```python
from build123d import *

# Parameters (mm, degrees)
F0_W     = 330.2
F0_H     = 533.4
F0_W_2   = 279.4
F0_H_2   = 482.6
F1_DEPTH = 381
F3_DEPTH = 11.43
F5_D     = 31.75
F6_W     = 330.2
F6_H     = 533.4
F7_DEPTH = 25.4


with BuildPart() as f1:
    # F0 (on Front) → F1 (new body)
    with BuildSketch(Plane.XZ):
        Rectangle(F0_W, F0_H)
        Rectangle(F0_W_2, F0_H_2, mode=Mode.SUBTRACT)
    extrude(amount=F1_DEPTH)

    # F2 (on face) → F3 (join)
    with BuildSketch(Plane.YZ.offset(165.1)):
        with BuildLine():
            add(Edge.make_bspline(
                [(-381, -6.6830463366), (-397.4427610563, -10.9233558088), (-440.2612759163, -2.0870202582), (-482.6984064218, 23.1422229449), (-443.5296874883, 46.3759759497), (-397.7583791554, 55.5903688255), (-381, 53.9625514371)],
                knots=[0.054305568, 0.054305568, 0.054305568, 0.054305568, 0.2287997299, 0.4012099815, 0.5729439025, 0.7296806034, 0.7296806034, 0.7296806034, 0.7296806034], degree=3))
            Line((-381, -6.6830463366), (-381, 53.9625514371))
        make_face()
        with BuildLine():
            add(Edge.make_bspline(
                [(-367.3923313618, 0), (-371.2589549432, -3.2025358081), (-375.8827314956, -5.3633894957), (-381, -6.6830463366)],
                knots=[0, 0, 0, 0, 0.054305568, 0.054305568, 0.054305568, 0.054305568], degree=3))
            add(Edge.make_bspline(
                [(-381, 53.9625514371), (-372.0113951219, 53.0894474703), (-347.8101498957, 44.708864678), (-354.1310052856, 10.9837098771), (-367.3923313618, 0)],
                knots=[0.7296806034, 0.7296806034, 0.7296806034, 0.7296806034, 0.8137486544, 1, 1, 1, 1], degree=3))
            Line((-381, 53.9625514371), (-381, -6.6830463366))
        make_face()
    extrude(amount=-F3_DEPTH)

    # F5 (through all)
    with Locations(Plane.YZ.offset(165.1)):
        with Locations((-419.4230139256, 24.0488089621)):
            Hole(F5_D / 2)

    # F6 (on face) → F7 (join)
    with BuildSketch(Plane(origin=(0, 0, 0), x_dir=(-1, 0, 0), z_dir=(0, 1, 0))):
        Rectangle(F6_W, F6_H)
    extrude(amount=F7_DEPTH)


solid = f1.part
```
Source: CAD feature listing. Evaluate the final solid. Frame: model axes, mm. A direction names the side the tool comes from. Coordinates: 2 decimals unless noted, no trailing zeros. Write each loop counter-clockwise with the first axis right and the second up, starting at its lowest first coordinate (ties: lowest second). Pieces come first, ordered by that corner, then holes. Notation, with made-up numbers: M 68.25,-28.5 L 97.25,-28.5 A22 ccw 97.25,-12.5 Z; hole C 81,-1 d4. An arc over 180 degrees is marked long. Answer as a JSON object with one key per item and string values.
1. Access query for faces 4 (the flat face through (-2, -188, -241.3)), 5 (the flat face through (2, -181, 266.7)), 6 (the flat face through (153.67, -420, 8)). Directions: +Z, -Z, +X, -X, +Y, -Y. A direction counts if a zero-diameter tool reaches every point of the face in a straight line with its end or side. Return the directions, or none.
Evaluation:
{"face 4": "-Y", "face 5": "+Z, +X, -X, +Y, -Y", "face 6": "+Z, -Z, -X, -Y"}
2. Ray query, L1, parallel to X at y = -235, z = -167.5; L2, parallel to Z at x = -102, y = -54; L3, parallel to Y at x = 46.5, z = -171.5. Return the intervals inside material, ascending.
Evaluation:
{"L1": "-165.1 to -139.7, 139.7 to 165.1", "L2": "-266.7 to -241.3, 241.3 to 266.7", "L3": "0 to 25.4"}
3. Cut plane C-C on x = -80. Output: boundary loops of the cut face in (y, z), plus the area to 3 significant figures.
Evaluation:
{"outline": "M -381,-266.7 L 25.4,-266.7 L 25.4,266.7 L -381,266.7 L -381,241.3 L 0,241.3 L 0,-241.3 L -381,-241.3 Z", "area": "32,900 mm^2"}
4. Contact query for flat-ended pins moving along their axis: P1, Ø19, axis at y = -439.5, z = 37.5, coming from the -X side; P2, Ø1, axis at x = 114.5, z = 162.5, coming from the -Y side. Output: stop coordinate, or through.
Evaluation:
{"P1": "x = 153.67", "P2": "y = 0"}
5. Cut plane A-A on z = -48. Output: boundary loops of the cut face in (x, y), plus the area to 3 significant figures.
Evaluation:
{"outline": "M -165.1,-381 L -139.7,-381 L -139.7,0 L 139.7,0 L 139.7,-381 L 165.1,-381 L 165.1,25.4 L -165.1,25.4 Z", "area": "27,700 mm^2"}
6. Draft query along X for faces 1 (the flat face through (2, -181, -266.7)), 2 (the flat face through (-165.1, -181, -4)), 3 (the flat face through (139.7, -188, -3)). Return one class per face: released by +X, released by -X, zero draft, split by the parting line, or undercut.
Evaluation:
{"face 1": "zero draft", "face 2": "released by -X", "face 3": "undercut"}
7. Cut plane B-B on y = -150. Output: boundary loops of the cut face in (x, z), plus the area to 3 significant figures.
Evaluation:
{"outline": "M -165.1,-266.7 L 165.1,-266.7 L 165.1,266.7 L -165.1,266.7 Z; hole M -139.7,-241.3 L 139.7,-241.3 L 139.7,241.3 L -139.7,241.3 Z", "area": "41,300 mm^2"}
